The model under review builds one solid part; all positions refer to its coordinate system, in mm. A direction names the side the tool comes from. Round coordinates to 2 decimals unless told otherwise and drop trailing zeros.
Item 1: Machinability: for faces 1 (the face through (-18, 18, 1.946)), 2 (the face through (12, -33, 5.132)), 3 (the face through (10.955, -30.913, 3.844)), 4 (the face through (-17.6, 17.6, -5.08)), 5 (the face through (11, -31, -4.937)), which of the approach directions +Z, -Z, +X, -X, +Y, -Y give a long, thin tool a straight path to every point of the face, cutting with its end or side? Answer none if there is none.
Item 2: Draft analysis for pull direction Y (two halves, no side actions). For faces 6 (the face through (-17, 17, 0)), 7 (the face through (-17.783, 17.983, -2.504)), 8 (the face through (-18, 19, -6.096)), state which applies: +Y half, -Y half, draft (parallel to the pull), parting line (faces both ways), or undercut.
Item 3: Add section A-A (z = -1.5). State how many separate pieces and enclosed holes the cut face has, plus the area to 3 significant figures.
Item 4: Clearance check with flat-ended pins moving along their axes: pin 1 Ø12 at (y, z) = (-29.5, -7) entering from +X; pin 2 Ø10 at (x, y) = (1, -20.5) entering from -Z; pin 3 Ø6 at (y, z) = (-20, 7) entering from -X; pin 4 Ø2 at (x, y) = (-15, 0) entering from -Z. State where each tip first meets the part, or that it passes through.
Item 5: To check wall thickness, follow L1, parallel to Z at x = 1, y = -3.5; L2, parallel to Y at x = -24, z = 0.75; L3, parallel to Z at x = -14, y = 12.5. State the ranges of each line that lie inside material, in increasing order.
```python
from build123d import *

# Parameters (mm, degrees)
F2_W      = 7.8210735228
F2_H      = 1.6869045794
F3_DEPTH  = 7.874
F5_DEPTH  = 5.842
F7_DEPTH  = 2.54
F8_W      = 7.2907346766
F8_H      = 1.9461095799
F9_DEPTH  = 5.08
F11_DEPTH = 5.08
F13_DEPTH = 1.016


with BuildPart() as f1:
    # F0 (on Top) → F1 (revolve)
    with BuildSketch(Plane.XY):
        Polygon((9.738479662, -15.3682792879), (-3.4222373906, 6.3731869042), (-5.6319757583, 22.0445621817), (-15.939033498, 16.113988769), (9.3961827512, -27.9174258268), (19.7350436062, -21.9685532335), align=None)
    revolve(axis=Axis((-3.2714253734, -5.9017185289, 0), (0.4987248594, -0.8667603559, 0)))

    # F2 (on face) → F3 (join)
    with BuildSketch(Plane(origin=(14.4050829924, -25.0353569234, 0), x_dir=(0.8667603559, 0.4987248594, 0), z_dir=(0.4987248594, -0.8667603559, 0))):
        with Locations((-5.9160405071, -4.0938784368)):
            Rectangle(F2_W, F2_H)
    extrude(amount=F3_DEPTH)

    # F4 (on face) → F5 (join)
    with BuildSketch(Plane.XY.offset(-3.2504261471)):
        Polygon((15.1675006282, -30.3816657685), (8.3885041579, -34.2822295615), (9.8147549245, -36.7609863326), (16.5937513949, -32.8604225396), align=None)
    extrude(amount=F5_DEPTH)

    # F6 (on face) → F7 (join)
    with BuildSketch(Plane.XY.offset(2.5915738529)):
        Polygon((9.8147549245, -36.7609863326), (16.5937513949, -32.8604225396), (14.2455248972, -29.0196318337), (7.5704112418, -32.8604225396), align=None)
    extrude(amount=F7_DEPTH)

    # F8 (on face) → F9 (join)
    with BuildSketch(Plane(origin=(-10.9301332567, 18.9960576725, 0), x_dir=(-0.8667603559, -0.4987248594, 0), z_dir=(-0.4987248594, 0.8667603559, 0))):
        with Locations((6.4960370073, 0.9730547899)):
            Rectangle(F8_W, F8_H)
    extrude(amount=F9_DEPTH)

    # F10 (on face) → F11 (join)
    with BuildSketch(Plane(origin=(0, 0, 0), x_dir=(1, 0, 0), z_dir=(0, 0, -1))):
        Polygon((-22.2538227827, -18.3414298242), (-15.9345029994, -21.9775004507), (-14.6677418565, -19.7759291467), (-20.9870616398, -16.1398585201), align=None)
    extrude(amount=F11_DEPTH)

    # F12 (on face) → F13 (join)
    with BuildSketch(Plane(origin=(0, 0, -5.08), x_dir=(1, 0, 0), z_dir=(0, 0, -1))):
        Polygon((-22.2538227827, -18.3414298242), (-15.9345029994, -21.9775004507), (-14.1230425955, -18.8292674424), (-20.4423623788, -15.1931968158), align=None)
    extrude(amount=F13_DEPTH)


solid = f1.part
```
Numbers:
1. face 1: +Z, -X, +Y
1. face 2: +Z, +X, -Y
1. face 3: +Z
1. face 4: none
1. face 5: -Z, +X, -Y
2. face 6: undercut
2. face 7: undercut
2. face 8: draft
3. separate pieces: 3
3. enclosed holes: 0
3. area: 804 mm2
4. pin 1: stops at x = 17.07
4. pin 2: stops at z = -8.76
4. pin 3: stops at x = -1.53
4. pin 4: passes through
5. L1: z = -3.85 to 3.85
5. L2: y = 8.45 to 11.48
5. L3: z = -10.24 to 10.24
